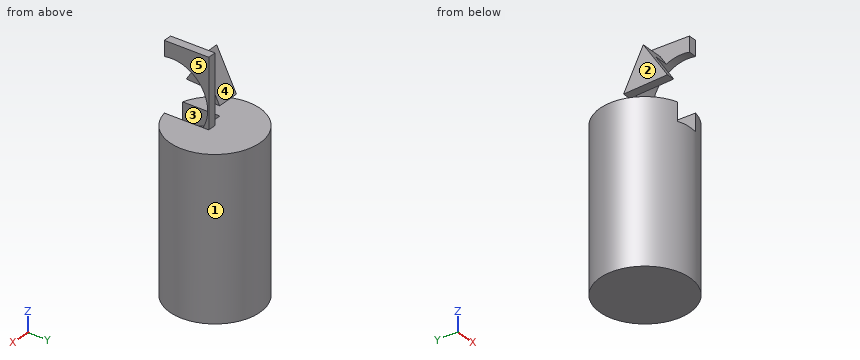
from build123d import *

# Parameters (mm, degrees)
F0_R     = 50.432717
F1_DEPTH = 177.8
F2_W     = 9.432334
F2_H     = 49.54281
F3_DEPTH = 76.2
F5_DEPTH = 25.4
F6_R     = 40.466301
F7_DEPTH = 25.4


with BuildPart() as f1:
    # F0 (on Top) → F1 (new body)
    with BuildSketch(Plane.XY):
        Circle(F0_R)
    extrude(amount=F1_DEPTH)

    # F2 (on face) → F3 (join)
    with BuildSketch(Plane.XY.offset(177.8)):
        with Locations((4.716167, -24.771405)):
            Rectangle(F2_W, F2_H)
    extrude(amount=F3_DEPTH)

    # F4 (on face) → F5 (join)
    with BuildSketch(Plane(origin=(0, 0, 0), x_dir=(0, -1, 0), z_dir=(-1, 0, 0))):
        Polygon((16.824646, 244.190742), (-5.220201, 200.336856), (43.780802, 203.172401), align=None)
    extrude(amount=F5_DEPTH)

    # F6 (on face) → F7 (cut)
    with BuildSketch(Plane.YZ.offset(9.432334)):
        with Locations((-41.694514, 197.413847)):
            Circle(F6_R)
    extrude(amount=-F7_DEPTH, mode=Mode.SUBTRACT)


solid = f1.part
Source: CAD feature listing. Evaluate the final solid. Frame: model axes, mm. Face numbers are marked on the shaded views. A direction names the side the tool comes from. Coordinates: 2 decimals unless noted, no trailing zeros. Write each loop counter-clockwise with the first axis right and the second up, starting at its lowest first coordinate (ties: lowest second). Pieces come first, ordered by that corner, then holes. Notation, with made-up numbers: M 49.5,7.25 L 56.5,7.25 A20 cw 56.5,13.25 Z; hole C 76,54.25 d4. An arc over 180 degrees is marked long. Use a Markdown table: item, result.
1) First-contact query: pin 1 Ø6 at (x, z) = (20, 161) entering from +Y; pin 2 Ø4.5 at (x, z) = (3, 248.5) entering from -Y; pin 3 Ø16.5 at (y, z) = (-16.5, 209.5) entering from +X; pin 4 Ø10 at (y, z) = (5, 149) entering from +X. Flat tips, straight axial feed; report the tip coordinate or a pass-through.
Conclusion:
| item | result |
|---|---|
| pin 1 | stops at y = 47.48 |
| pin 2 | stops at y = -49.54 |
| pin 3 | stops at x = -15.97 |
| pin 4 | stops at x = 50.43 |
2) Section C-C, the plane x = -22. Output: boundary loops of the cut face in (y, z), then the cut area to 3 significant figures.
Conclusion:
| item | result |
|---|---|
| outline | M -45.38,0 L 45.38,0 L 45.38,177.8 L -45.38,177.8 Z; M -43.78,203.17 L 5.22,200.34 L -16.82,244.19 Z |
| area | 17,200 mm^2 |
3) Section B-B, the plane z = 228. Output: boundary loops of the cut face in (x, y).
Conclusion:
| item | result |
|---|---|
| outline | M -25.4,-27.46 L -15.97,-27.46 L -15.97,-15.2 L 9.43,-15.2 L 9.43,0 L 0,0 L 0,-8.69 L -25.4,-8.69 Z |
4) Section A-A, the plane y = -37. Output: boundary loops of the cut face in (x, z).
Conclusion:
| item | result |
|---|---|
| outline | M -34.27,0 L 34.27,0 L 34.27,177.8 L 9.43,177.8 L 9.43,157.22 L -15.97,157.22 L -15.97,177.8 L -34.27,177.8 Z; M -25.4,202.78 L -15.97,202.78 L -15.97,213.49 L -25.4,213.49 Z; M 0,237.61 L 9.43,237.61 L 9.43,254 L 0,254 Z |
5) Section D-D, the plane x = 39. Output: boundary loops of the cut face in (y, z), then the cut area to 3 significant figures.
Conclusion:
| item | result |
|---|---|
| outline | M -31.98,0 L 31.98,0 L 31.98,177.8 L -31.98,177.8 Z |
| area | 11,400 mm^2 |
6) Reachability of the marked faces 1 and 2 from +Z, -Z, +X, -X, +Y, -Y: full face, straight path, thin tool, end or side. Return the list, or none.
Conclusion:
| item | result |
|---|---|
| face 1 | +Z, -Z |
| face 2 | +Z, -X, +Y, -Y |
7) Mould query, pull axis Z, two halves, no side actions, for the marked faces 3, 4 and 5. Classes: pulls with the +Z half, pulls with the -Z half, needs draft (parallel to the pull), parting line crosses it, or undercut.
Conclusion:
| item | result |
|---|---|
| face 3 | undercut |
| face 4 | pulls with the +Z half |
| face 5 | needs draft |
8) Ray query, L1, parallel to Z at x = 1, y = 30.5; L2, parallel to X at y = 0.5, z = 31; L3, parallel to Z at x = -23.5, y = -16. Return the intervals inside material, ascending.
Conclusion:
| item | result |
|---|---|
| L1 | z = 0 to 177.8 |
| L2 | x = -50.43 to 50.43 |
| L3 | z = 0 to 177.8, 201.56 to 242.55 |
